Check sheet for the modelled part. Datum: model origin and axes. Units: mm. A direction names the side the tool comes from. Round coordinates to 2 decimals unless told otherwise and drop trailing zeros. Write each loop counter-clockwise with the first axis right and the second up, starting at its lowest first coordinate (ties: lowest second). Pieces come first, ordered by that corner, then holes. Notation, with made-up numbers: M -35,32 L -16,32 A14 ccw -16,45 Z; hole C -2.5,-27 d6. An arc over 180 degrees is marked long. Answer in a Markdown table with one row per item.
```python
from build123d import *

# Parameters (mm, degrees)
SKETCH1_R           = 5.25
BOSS_EXTRUDE1_DEPTH = 2.5
BOSS_EXTRUDE2_DEPTH = 2.3


with BuildPart() as part:
    # Sketch1 → Boss-Extrude1 (new body)
    with BuildSketch(Plane(origin=(0, 0, 0), x_dir=(1, 0, 0), z_dir=(0, 1, 0))):
        with BuildLine():
            ThreePointArc((6.154078518, -12.360831122), (11.656426966, -7.310595529), (13.692219593, -0.124757626))
            ThreePointArc((13.692219593, -0.124757626), (-5.843155784, 12.270337945), (-8.736743065, -10.683886895))
            ThreePointArc((-8.736743065, -10.683886895), (-1.238774651, -11.05566121), (6.154078518, -12.360831122))
        make_face()
        with Locations((-0.007780407, -0.124757626)):
            Circle(SKETCH1_R, mode=Mode.SUBTRACT)
    extrude(amount=BOSS_EXTRUDE1_DEPTH)

    # Sketch2 → Boss-Extrude2 (add)
    with BuildSketch(Plane(origin=(0, 2.5, 0), x_dir=(1, 0, 0), z_dir=(0, 1, 0))):
        with BuildLine():
            ThreePointArc((6.154078518, -12.360831122), (-1.238774651, -11.05566121), (-8.736743065, -10.683886895))
            ThreePointArc((-8.736743065, -10.683886895), (1.52536697, 13.489185929), (6.154078518, -12.360831122))
        make_face()
    extrude(amount=BOSS_EXTRUDE2_DEPTH)


solid = part.part
```
1. Section check C-C, the plane y = 1.85. Record the cut outline in (x, z).
Found:
| item | result |
|---|---|
| outline | M -8.74,10.68 A13.7 ccw long 6.15,12.36 A60 cw Z; hole C -0.01,0.12 d10.5 |
2. Go/stop test with flat-tipped pins: pin 1 (1 mm diameter, centred on y = 2, z = -10.5, fed in from +X); pin 2 (1.5 mm diameter, centred on y = 1.5, z = -7, fed in from -X); pin 3 (2 mm diameter, centred on y = 3.5, z = 3, fed in from -X). Record where each tip stops, or that it passes through.
Found:
| item | result |
|---|---|
| pin 1 | stops at x = 9.22 |
| pin 2 | stops at x = -12.13 |
| pin 3 | stops at x = -13.58 |
3. Section check B-B, the plane z = 6.5. Record the cut outline in (x, y), and give its area (3 significant figures).
Found:
| item | result |
|---|---|
| outline | M -12.13,0 L 12.12,0 L 12.12,4.8 L -12.13,4.8 Z |
| area | 116 mm2 |
4. Access from +Z, -Z, +X, -X, +Y, -Y to the whole of each face (thin tool, end or side, straight path). Record for faces 1 (the face through (0, 4.8, -1)), 2 (the face through (0, 2.5, 0)).
Found:
| item | result |
|---|---|
| face 1 | +Z, -Z, +X, -X, +Y |
| face 2 | -Y |
5. Scan lines: L1, parallel to Y at x = -1.75, z = 2.75; L2, parallel to Z at x = 4.75, y = 2.1; L3, parallel to Z at x = -3.75, y = 1.05. Record each from-to range of solid material in increasing order.
Found:
| item | result |
|---|---|
| L1 | y = 2.5 to 4.8 |
| L2 | z = -12.72 to -2.09, 2.34 to 12.04 |
| L3 | z = -13.05 to -3.56, 3.81 to 10.83 |
6. Draft check along Z on faces 3 (the face through (5, 1.23, -1.45)), 4 (the face through (6, 0, -1)), 5 (the face through (-1.13, 2.37, 11.07)). Enter one of: +Z half, -Z half, draft (parallel to the pull), parting line (faces both ways), or undercut.
Found:
| item | result |
|---|---|
| face 3 | undercut |
| face 4 | draft |
| face 5 | +Z half |
7. Section check D-D, the plane y = 3.9. Record the cut outline in (x, z), and give its area (3 significant figures).
Found:
| item | result |
|---|---|
| outline | M -8.74,10.68 A13.7 ccw long 6.15,12.36 A60 cw Z |
| area | 562 mm2 |
8. Section check A-A, the plane x = 1. Record the cut outline in (y, z), and give its area (3 significant figures).
Found:
| item | result |
|---|---|
| outline | M 0,-13.54 L 4.8,-13.54 L 4.8,11.35 L 0,11.35 L 0,5.28 L 2.5,5.28 L 2.5,-5.03 L 0,-5.03 Z |
| area | 93.7 mm2 |
